from build123d import *

# Parameters (mm, degrees)
BOSS_EXTRUDE1_DEPTH = 6.35
SKETCH4_R           = 2.0828
SKETCH4_R_2         = 2.2225
CUT_EXTRUDE1_DEPTH  = 50.8
SKETCH5_W           = 7.9375
SKETCH5_H           = 12.7
CUT_EXTRUDE2_DEPTH  = 6.35
FILLET1_R           = 3.175


with BuildPart() as part:
    # Sketch3 → Boss-Extrude1 (new body)
    with BuildSketch(Plane(origin=(0, 0, 0), x_dir=(1, 0, 0), z_dir=(0, 1, 0))):
        Polygon((55.304809527, 7.379629834), (47.367309527, 7.379629834), (47.367309527, -11.670370166), (72.767309527, -11.670370166), (72.767309527, 7.379629834), (68.004809527, 7.379629834), align=None)
        Polygon((26.729809527, 7.379629834), (39.429809527, 7.379629834), (39.429809527, 13.729629834), align=None)
        Polygon((55.304809527, 13.729629834), (55.304809527, 7.379629834), (68.004809527, 7.379629834), align=None)
        Polygon((47.367309527, -11.670370166), (47.367309527, 7.379629834), (39.429809527, 7.379629834), (26.729809527, 7.379629834), (21.967309527, 7.379629834), (21.967309527, -11.670370166), align=None)
        Polygon((55.304809527, 39.129629834), (47.367309527, 39.129629834), (47.367309527, 7.379629834), (55.304809527, 7.379629834), (55.304809527, 13.729629834), align=None)
        Polygon((47.367309527, 7.379629834), (47.367309527, 39.129629834), (39.429809527, 39.129629834), (39.429809527, 13.729629834), (39.429809527, 7.379629834), align=None)
    extrude(amount=BOSS_EXTRUDE1_DEPTH)

    # Sketch4 → Cut-Extrude1 (cut)
    with BuildSketch(Plane(origin=(55.304809527, 0, 0), x_dir=(0, 0, -1), z_dir=(1, 0, 0))):
        with Locations((21.667129834, 3.175)):
            Circle(SKETCH4_R)
        with Locations((34.367129834, 3.175)):
            Circle(SKETCH4_R_2)
    extrude(amount=-CUT_EXTRUDE1_DEPTH, mode=Mode.SUBTRACT)

    # Sketch5 → Cut-Extrude2 (cut)
    with BuildSketch(Plane(origin=(0, 6.35, 0), x_dir=(1, 0, 0), z_dir=(0, 1, 0))):
        with Locations((51.336059527, 32.779629834)):
            Rectangle(SKETCH5_W, SKETCH5_H)
    extrude(amount=-CUT_EXTRUDE2_DEPTH, mode=Mode.SUBTRACT)

    # Fillet1
    fillet1_edges = [part.edges().sort_by_distance(p)[0] for p in [
        (51.336059527, 6.35, -26.429629834),
    ]]
    fillet(fillet1_edges, radius=FILLET1_R)


solid = part.part
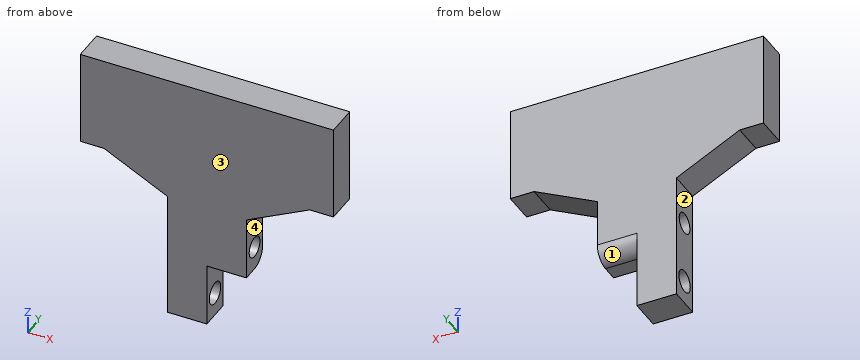
Verification items for the finished model (mm, model axes). Face numbers are marked on the shaded views. A direction names the side the tool comes from. Give positions to 0.01 mm unless a question says otherwise; leave off trailing zeros. Loops run counter-clockwise (first coordinate to the right, second up) from the corner with the lowest first, then second, coordinate; pieces in that order, holes last.
1. Go/stop test with flat-tipped pins: P1, Ø3.5, axis at x = 50.5, y = 1.5, coming from the -Z side; P2, Ø2.5, axis at x = 25, y = 4, coming from the -Z side; P3, Ø3, axis at y = 3.5, z = -26.5, coming from the -X side. Record where each tip stops, or that it passes through.
Derived:
P1: stops at z = -26.43
P2: stops at z = -7.38
P3: stops at x = 39.43
2. Cross-section at D-D on z = -30. Record the cut outline in (x, y), and give its area (3 significant figures).
Derived:
outline: (39.43, 0) - (47.37, 0) - (47.37, 6.35) - (39.43, 6.35) - close
area: 50.4 mm2
3. Cross-section at B-B on y = 2. Record the cut outline in (x, z), and give its area (3 significant figures).
Derived:
outline: (21.97, -7.38) - (26.73, -7.38) - (39.43, -13.73) - (39.43, -19.95) - (55.3, -19.95) - (55.3, -13.73) - (68, -7.38) - (72.77, -7.38) - (72.77, 11.67) - (21.97, 11.67) - close; (39.43, -39.13) - (47.37, -39.13) - (47.37, -36.25) - (39.43, -36.25) - close; (39.43, -32.48) - (47.37, -32.48) - (47.37, -26.43) - (55.3, -26.43) - (55.3, -23.39) - (39.43, -23.39) - close
area: 1,370 mm2
4. Tool access check on the marked faces 1, 2, 3 and 4. Record the directions out of +Z, -Z, +X, -X, +Y, -Y that give a thin tool (end or side, any length) a straight path to the whole face; none if there is none.
Derived:
face 1: -Z, +X, +Y
face 2: -Z, -X, +Y, -Y
face 3: +Z, -Z, +X, -X, -Y
face 4: -Z, +X, +Y, -Y
5. Cross-section at C-C on x = 54.5. Record the cut outline in (y, z) (3 decimals), and give its area (3 significant figures).
Derived:
outline: (0, -26.43) - (3.175, -26.43) arc R3.175 ccw to (6.35, -23.255) - (6.35, 11.67) - (0, 11.67) - close; hole circle Ø4.166 at (3.175, -21.667)
area: 226 mm2
6. Material ranges on probe 1 along Z at (x, y) = (55, 3.25); probe 2 along Z at (x, y) = (46, 4); probe 3 along Z at (x, y) = (39.5, 3.5), recorded low to high.
Derived:
probe 1: z = -26.43 to -23.75, -19.59 to 11.67
probe 2: z = -39.13 to -36.43, -32.3 to -23.58, -19.75 to 11.67
probe 3: z = -39.13 to -36.57, -32.17 to -23.72, -19.61 to 11.67
7. Cross-section at A-A on x = 43. Count the separate pieces of the cut face and the enclosed holes in it, and give its area (3 significant figures).
Derived:
separate pieces: 1
enclosed holes: 2
area: 293 mm2
